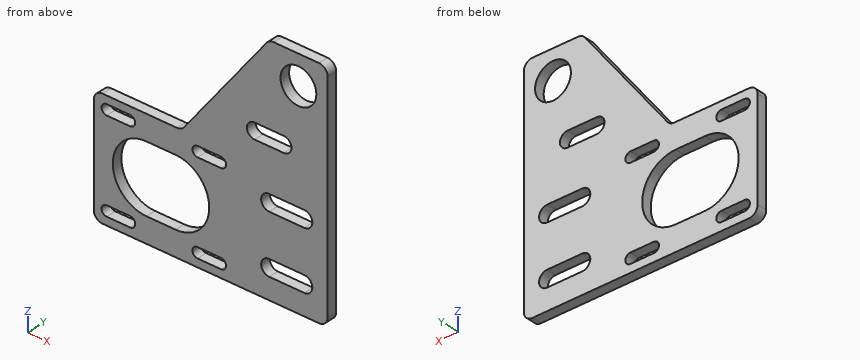
Autodesk Inventor part; units mm, degrees
ref_plane "YZ Plane" through (0, 0, 0) normal (1, 0, 0) x (0, 1, 0)
ref_plane "XZ Plane" through (0, 0, 0) normal (0, 1, 0) x (-1, 0, 0)
ref_plane "XY Plane" through (0, 0, 0) normal (0, 0, 1) x (1, 0, 0)
sketch "Sketch1" plane through (0, 0, 0) normal (0, 1, 0) x (-1, 0, 0)
  line L0 (-40, 40) -> (40, 40)
  line L1 (40, 40) -> (40, -40)
  line L2 (40, -40) -> (-40, -40)
  line L3 (-40, -40) -> (-40, 40)
  point P0 (0, 0)
  dimension "d0" = 80
  dimension "d1" = 80
  dimension "d2" = 40
  dimension "d3" = 40
extrude "Extrusion1" add sketch "Sketch1" along normal blind 3.4163
sketch "Sketch2" plane through (0, 3.4163, 0) normal (0, 1, 0) x (1, 0, 0)
  line L0 (40, -40) -> (40, 40)
  line L1 (40, 40) -> (-40, 40)
  arc A0 (20, 32.75) -> (20, 27.25) centre (20, 30) ccw
  arc A1 (20, 12.75) -> (20, 7.25) centre (20, 10) ccw
  line L2 (20, 32.75) -> (32, 32.75)
  line L3 (20, 27.25) -> (32, 27.25)
  line L4 (20, 12.75) -> (32, 12.75)
  line L5 (20, 7.25) -> (32, 7.25)
  arc A2 (32, 27.25) -> (32, 32.75) centre (32, 30) ccw
  arc A3 (32, 7.25) -> (32, 12.75) centre (32, 10) ccw
  point P0 (0, 0)
  point P1 (40, 32.75)
  point P2 (40, 27.25)
  point P3 (40, 12.75)
  point P4 (40, 7.25)
  dimension "d6" = 5.5
  dimension "d7" = 5.5
  dimension "d8" = 20
  dimension "d9" = 10
  dimension "d10" = 20
  dimension "d11" = 20
  dimension "d72" = 5.5
  dimension "d73" = 10
  dimension "d74" = 8
  dimension "d75" = 5.5
  dimension "d76" = 20
  dimension "d77" = 8
extrude "Extrusion2" cut sketch "Sketch2" against normal through all
sketch "Sketch3" plane through (0, 3.4163, 0) normal (0, 1, 0) x (1, 0, 0)
  line L0 (40, 40) -> (-40, 40)
  line L1 (40, -40) -> (40, 40)
  circle A0 centre (30, -30) radius 6.125
  point P0 (40, 7.25)
  point P1 (0, 0)
  dimension "d14" = 12.25
  dimension "d15" = 10
  dimension "d16" = 70
extrude "Extrusion3" cut sketch "Sketch3" against normal through all
sketch "Sketch4" plane through (0, 3.4163, 0) normal (0, 1, 0) x (1, 0, 0)
  line L0 (40, 40) -> (-40, 40)
  line L1 (-40, 40) -> (-40, -40)
  line L2 (-40, -40) -> (40, -40)
  line L3 (32, 27.25) -> (20, 27.25)
  line L4 (-40, 0) -> (-10, 0)
  line L5 (-10, 0) -> (20, -40)
  point P0 (40, 27.25)
  point P1 (0, 0)
  dimension "d19" = 30
  dimension "d21" = 40
  dimension "d22" = 60
extrude "Extrusion4" cut sketch "Sketch4" against normal through all
fillet "Fillet1" radius 3 6 edges at (40, 1.7082, 40) (20, 1.7082, 40) (40, 1.7082, -40) (-10, 1.7082, 0) (-40, 1.7082, 0) (-40, 1.7082, -40)
sketch "Sketch5" plane through (0, 3.4163, 0) normal (0, 1, 0) x (1, 0, 0)
  line L0 (40, -37) -> (40, 37)
  line L1 (37, 40) -> (-37, 40)
  arc A0 (-12, 8.5) -> (-12, 31.5) centre (-12, 20) ccw
  line L2 (-12, 31.5) -> (-22, 31.5)
  line L3 (-12, 8.5) -> (-22, 8.5)
  arc A1 (-22, 31.5) -> (-22, 8.5) centre (-22, 20) ccw
  point P0 (40, 15.75)
  point P1 (40, 24.25)
  point P2 (0, 0)
  dimension "d26" = 23
  dimension "d27" = 52
  dimension "d35" = 23
  dimension "d36" = 10
  dimension "d37" = 10
  dimension "d38" = 20
  dimension "d39" = 20
  dimension "d42" = 52
  dimension "d81" = 8.5
  dimension "d82" = 8.5
extrude "Extrusion5" cut sketch "Sketch5" against normal through all
sketch "Sketch6" plane through (0, 3.4163, 0) normal (0, 1, 0) x (1, 0, 0)
  line L0 (40, -37) -> (40, 37)
  line L1 (37, 40) -> (-37, 40)
  arc A0 (3.5, 33.75) -> (3.5, 37.25) centre (3.5, 35.5) ccw
  arc A1 (-4.5, 37.25) -> (-4.5, 33.75) centre (-4.5, 35.5) ccw
  line L2 (-4.5, 37.25) -> (3.5, 37.25)
  line L3 (3.5, 33.75) -> (-4.5, 33.75)
  point P0 (40, 35.75)
  point P1 (0, 0)
  dimension "d48" = 3.5
  dimension "d49" = 4.5
  dimension "d50" = 36.5
  dimension "d51" = 3.5
  dimension "d52" = 4.5
  dimension "d53" = 44.5
  dimension "d78" = 8
extrude "Extrusion6" cut sketch "Sketch6" against normal through all
pattern_linear "Rectangular Pattern1" count 2 spacing 31.1 along (-1, 0, 0) count 2 spacing 31.1 along (0, 0, 1) of "Extrusion6"
sketch "Sketch7" plane through (0, 3.4163, 0) normal (0, 1, 0) x (1, 0, 0)
  line L0 (21.5, -40) -> (37, -40)
  line L1 (40, -37) -> (40, 37)
  arc A0 (25, -12.625) -> (25, -7.375) centre (25, -10) ccw
  arc A1 (15, -7.375) -> (15, -12.625) centre (15, -10) ccw
  line L2 (15, -7.375) -> (25, -7.375)
  line L3 (25, -12.625) -> (15, -12.625)
  point P0 (40, 4.25)
  point P1 (0, 0)
  dimension "d63" = 5.25
  dimension "d64" = 15
  dimension "d65" = 30
  dimension "d66" = 5.25
  dimension "d67" = 10
  dimension "d68" = 30
  dimension "d69" = 10
extrude "Extrusion7" cut sketch "Sketch7" against normal through all
equation "\"d73\" = d9"
equation "\"d76\" = d8"
equation "\"d77\" = d74"
equation "\"d35\" = d26"
equation "\"d42\" = d27"
equation "\"d66\" = d63"
properties part number "z_motor_mount_plate"
Model file for the job. Use its own axes, mm. Round coordinates to 2 decimals unless told otherwise and drop trailing zeros. Order: outer loops, then holes, each group sorted by start corner. A loop starts at its lowest first (then second) coordinate and runs counter-clockwise, first axis right, second up. Notation, with made-up numbers: M 56.25,9.25 L 93.25,9.25 A19 cw 93.25,27.25 Z; hole C -30.5,38 d5. An arc over 180 degrees is marked long. Write each question's results on one line, items separated by ' | '. Start each with the question number.
(1) Saw through at B-B, the plane x = 13.5. Give the cut face in (y, z), then the cut area to 3 significant figures.
(2) Saw through at A-A, the plane z = 10. Give the cut face in (x, y) (3 decimals).
(3) Probe probe 1 along X at (y, z) = (2.2, -11.5); probe 2 along X at (y, z) = (2.8, -34); probe 3 along Z at (x, y) = (26, 1.1). List the from-to ranges inside material, lowest first. Write a range as from..to.
(4) Drop flat-ended pins along their axis: pin 1 (6 mm diameter, centred on x = -15, z = -13, fed in from +Y); pin 2 (1 mm diameter, centred on x = -2, y = 2.5, fed in from +Z); pin 3 (1.7 mm diameter, centred on x = -33, y = 2, fed in from +Z). Give the stop position or say it passes through.
(5) Saw through at C-C, the plane z = -35.5. Give the cut face in (x, y), then the cut area to 3 significant figures.
(6) Saw through at D-D, the plane y = 1.65. State how many separate pieces and enclosed holes the cut face has, then the cut area to 3 significant figures.
Established:
1) outline: M 0,-40 L 3.42,-40 L 3.42,7.85 L 0,7.85 Z; M 0,12.15 L 3.42,12.15 L 3.42,31.33 L 0,31.33 Z | area: 229 mm^2
2) outline: M -2.5,0 L 12.375,0 L 12.375,3.416 L -2.5,3.416 Z; M 27.625,0 L 40,0 L 40,3.416 L 27.625,3.416 Z
3) probe 1: x = -40..-29.75, -4.25..17.7, 34.3..40 | probe 2: x = -40..-36.5, -26.7..-5.4, 4.4..40 | probe 3: z = -40..-32.75, -27.25..-12.75, -7.25..7.57, 12.43..25.36, 34.64..40
4) pin 1: passes through | pin 2: stops at z = 11.33 | pin 3: stops at z = 0
5) outline: M -40,0 L -37.35,0 L -37.35,3.42 L -40,3.42 Z; M -25.85,0 L -6.25,0 L -6.25,3.42 L -25.85,3.42 Z; M 5.25,0 L 40,0 L 40,3.42 L 5.25,3.42 Z | area: 195 mm^2
6) separate pieces: 1 | enclosed holes: 9 | area: 3,420 mm^2
